Can you work these out from the drawing? Everything is in mm from the part's minimum corner. A direction names the side the tool comes from. Coordinates: 2 decimals unless noted, no trailing zeros. Write each loop counter-clockwise with the first axis right and the second up, starting at its lowest first coordinate (ties: lowest second). Pieces come first, ordered by that corner, then holes.
(1) Please list where these lines run through material, in increasing order: probe 1 along X at (y, z) = (82, 125); probe 2 along Y at (x, z) = (64, 35); probe 3 along Z at (x, y) = (139, 75).
(2) For pin 1 Ø4 at (x, y) = (72.5, 68.5) entering from -Z; pin 2 Ø6 at (x, z) = (195.5, 42) entering from +Y; pin 3 Ø6 at (x, y) = (180.5, 40.5) entering from -Z, each with a flat end and sliding along its axis, tell me the tip position at first contact or that it passes through.
(3) Imagine slicing it at D-D, the plane z = 188.5. List the corners of the cut face in (x, y) for me.
(4) Thinking about a two-plate mould opening in X: for the marked faces 1 and 2, which applies, released by +X, released by -X, zero draft, split by the parting line, or undercut?
(5) Imagine slicing it at C-C, the plane y = 81. List the corners of the cut face in (x, z) for me, plus the area to 3 significant figures.
(6) Which directions (+Z, -Z, +X, -X, +Y, -Y) give clear straight access to the entire face, cutting with the end or side of a thin tool? Please do the marked faces 3, 4, 5, 6 and 7.
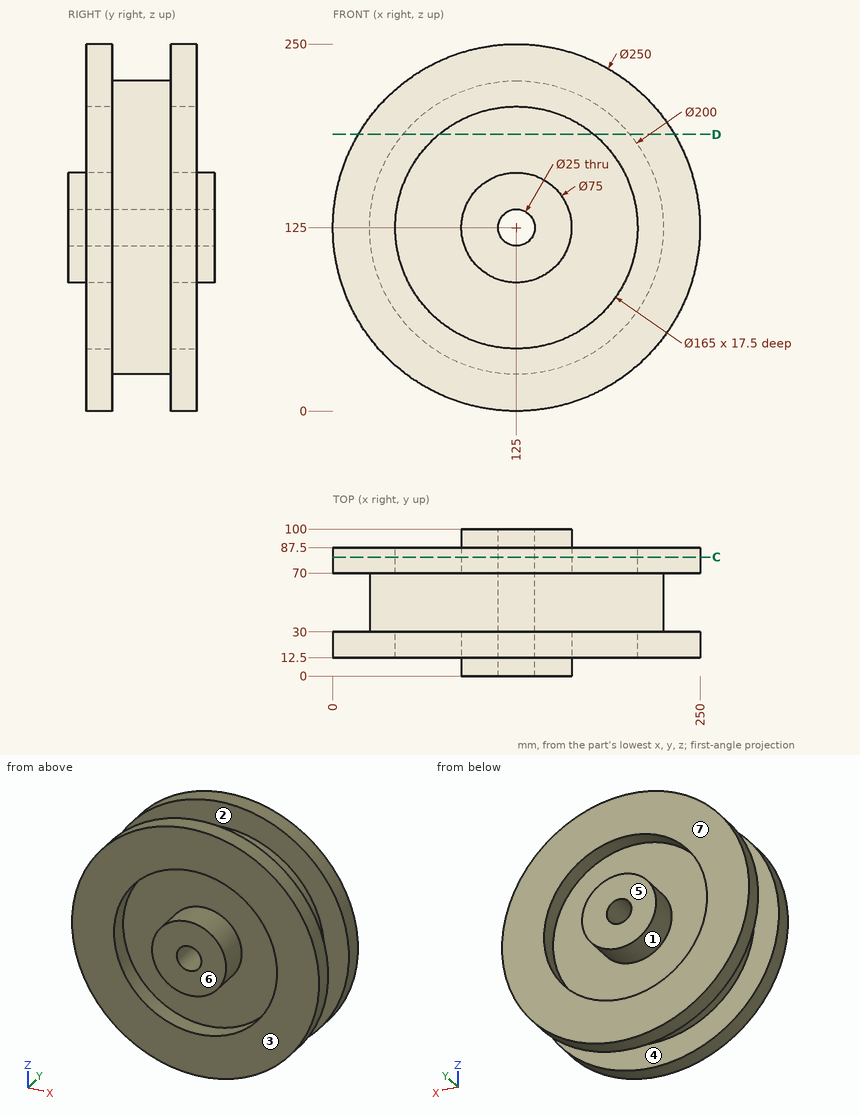
Recorded:
1. probe 1: x = 0 to 42.5, 87.5 to 112.5, 137.5 to 162.5, 207.5 to 250
1. probe 2: y = 12.5 to 30, 70 to 87.5
1. probe 3: z = 0.79 to 43.7, 90.21 to 159.79, 206.3 to 249.21
2. pin 1: stops at z = 10.96
2. pin 2: stops at y = 87.5
2. pin 3: stops at z = 39.89
3. outline: (17.33, 12.5) - (72.33, 12.5) - (72.33, 30) - (177.67, 30) - (177.67, 12.5) - (232.67, 12.5) - (232.67, 30) - (202.25, 30) - (202.25, 70) - (232.67, 70) - (232.67, 87.5) - (177.67, 87.5) - (177.67, 70) - (72.33, 70) - (72.33, 87.5) - (17.33, 87.5) - (17.33, 70) - (47.75, 70) - (47.75, 30) - (17.33, 30) - close
4. face 1: undercut
4. face 2: zero draft
5. outline: circle Ø250 at (125, 125); circle Ø75 at (125, 125); hole circle Ø165 at (125, 125); hole circle Ø25 at (125, 125)
5. area: 31,600 mm2
6. face 3: -Y
6. face 4: none
6. face 5: +Z, -Z, +X, -X, +Y
6. face 6: +Z, -Z, +X, -X, -Y
6. face 7: +Y
